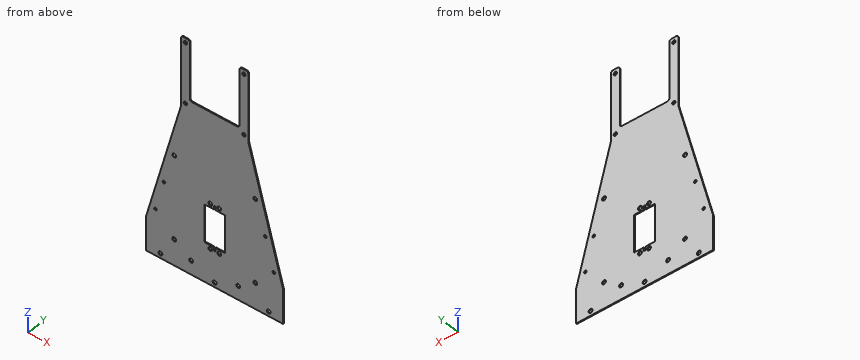
```python
from build123d import *

# Parameters (mm, degrees)
SKETCH26_R          = 1.875
SKETCH26_R_2        = 2.15
SKETCH26_R_3        = 1.45
BOSS_EXTRUDE6_DEPTH = 1


with BuildPart() as part:
    # Sketch26 → Boss-Extrude6 (new body)
    with BuildSketch(Plane(origin=(0, 0, 0), x_dir=(1, 0, 0), z_dir=(0, 1, 0))):
        with BuildLine():
            Line((76.013272408, 51.623832483), (76.013272408, 88.823544949))
            Line((76.013272408, 88.823544949), (-76.102081629, 88.823544949))
            Line((-76.102081629, 88.823544949), (-76.102081629, 51.776273242))
            Line((-76.102081629, 51.776273242), (-37.685470178, -85.312264175))
            ThreePointArc((-37.685470178, -85.312264175), (-37.546584556, -85.980512893), (-37.5, -86.661450073))
            Line((-37.5, -86.661450073), (-37.5, -159.216442532))
            ThreePointArc((-37.5, -159.216442532), (-36.767766953, -160.984209485), (-35, -161.716442532))
            Line((-35, -161.716442532), (-30, -161.716442532))
            ThreePointArc((-30, -161.716442532), (-28.232405329, -160.98438175), (-27.500000047, -159.216929795))
            Line((-27.500000047, -159.216929795), (-27.488305541, -99.215955269))
            ThreePointArc((-27.488305541, -99.215955269), (-26.755900259, -97.448503314), (-24.988305588, -96.716442532))
            Line((-24.988305588, -96.716442532), (24.988305588, -96.716442532))
            ThreePointArc((24.988305588, -96.716442532), (26.756072541, -97.448675579), (27.488305588, -99.216442532))
            Line((27.488305588, -99.216442532), (27.488305588, -159.216442532))
            ThreePointArc((27.488305588, -159.216442532), (28.220538635, -160.984209485), (29.988305588, -161.716442532))
            Line((29.988305588, -161.716442532), (34.988305588, -161.716442532))
            ThreePointArc((34.988305588, -161.716442532), (36.756072541, -160.984209485), (37.488305588, -159.216442532))
            Line((37.488305588, -159.216442532), (37.488305588, -86.69785128))
            ThreePointArc((37.488305588, -86.69785128), (37.534787412, -86.017661841), (37.673368657, -85.350118981))
            Line((37.673368657, -85.350118981), (75.502125614, 49.797698633))
            Line((75.502125614, 49.797698633), (76.013272408, 51.623832483))
        make_face()
        with Locations(Location((-32.5, -156.716442532, 0), (0, 0, 270))):
            Circle(SKETCH26_R, mode=Mode.SUBTRACT)
        with Locations(Location((-32.5, -91.716442532, 0), (0, 0, 270))):
            Circle(SKETCH26_R, mode=Mode.SUBTRACT)
        with Locations(Location((32.488305588, -156.716442532, 0), (0, 0, 270))):
            Circle(SKETCH26_R, mode=Mode.SUBTRACT)
        with Locations(Location((32.488305588, -91.716442532, 0), (0, 0, 270))):
            Circle(SKETCH26_R, mode=Mode.SUBTRACT)
        with Locations(Location((-44.91002895, -29.282587791, 0), (0, 0, 270))):
            Circle(SKETCH26_R_2, mode=Mode.SUBTRACT)
        with Locations(Location((-56.275133419, 5.22710987, 0), (0, 0, 270))):
            Circle(SKETCH26_R_3, mode=Mode.SUBTRACT)
        with Locations(Location((-4.91002895, 1.717412209, 0), (0, 0, 270))):
            Circle(SKETCH26_R_2, mode=Mode.SUBTRACT)
        with Locations(Location((-65.710275059, 38.931384113, 0), (0, 0, 270))):
            Circle(SKETCH26_R_3, mode=Mode.SUBTRACT)
        with Locations(Location((-60.263272408, 83.747616616, 0), (0, 0, 270))):
            Circle(SKETCH26_R_2, mode=Mode.SUBTRACT)
        with Locations(Location((-44.91002895, 60.717412209, 0), (0, 0, 270))):
            Circle(SKETCH26_R_2, mode=Mode.SUBTRACT)
        with Locations(Location((-4.91002895, 50.217412209, 0), (0, 0, 270))):
            Circle(SKETCH26_R_2, mode=Mode.SUBTRACT)
        with Locations(Location((-26.102081629, 73.823544949, 0), (0, 0, 270))):
            Circle(SKETCH26_R_2, mode=Mode.SUBTRACT)
        with Locations(Location((5.08997105, 1.717412209, 0), (0, 0, 270))):
            Circle(SKETCH26_R_2, mode=Mode.SUBTRACT)
        Polygon((11.577692982, 46.217412209), (11.577692982, 5.717412209), (1.08997105, 5.717412209), (1.08997105, 1.717412209), (-0.91002895, 1.717412209), (-0.91002895, 5.717412209), (-11.397750883, 5.717412209), (-11.397750883, 46.217412209), (-0.91002895, 46.217412209), (-0.91002895, 50.217412209), (1.08997105, 50.217412209), (1.08997105, 46.217412209), align=None, mode=Mode.SUBTRACT)
        with Locations(Location((45.08997105, -29.282587791, 0), (0, 0, 270))):
            Circle(SKETCH26_R_2, mode=Mode.SUBTRACT)
        with Locations(Location((56.276531408, 5.226515161, 0), (0, 0, 270))):
            Circle(SKETCH26_R_3, mode=Mode.SUBTRACT)
        with Locations(Location((5.08997105, 50.217412209, 0), (0, 0, 270))):
            Circle(SKETCH26_R_2, mode=Mode.SUBTRACT)
        with Locations(Location((0, 83.74802142, 0), (0, 0, 270))):
            Circle(SKETCH26_R_2, mode=Mode.SUBTRACT)
        with Locations(Location((26.102081629, 73.823544949, 0), (0, 0, 270))):
            Circle(SKETCH26_R_2, mode=Mode.SUBTRACT)
        with Locations(Location((65.7106575, 38.931073679, 0), (0, 0, 270))):
            Circle(SKETCH26_R_3, mode=Mode.SUBTRACT)
        with Locations(Location((45.08997105, 60.717412209, 0), (0, 0, 270))):
            Circle(SKETCH26_R_2, mode=Mode.SUBTRACT)
        with Locations(Location((59.999999999, 83.747618385, 0), (0, 0, 270))):
            Circle(SKETCH26_R_2, mode=Mode.SUBTRACT)
    extrude(amount=BOSS_EXTRUDE6_DEPTH)


solid = part.part
```
Here's how the part is built. I have some questions about the finished solid (model axes, mm). Coordinates: 2 decimals unless noted, no trailing zeros. Order: outer loops, then holes, each group sorted by start corner. A loop starts at its lowest first (then second) coordinate and runs counter-clockwise, first axis right, second up. Notation, with made-up numbers: (67, -12) -> (106, -12) arc R17 cw to (106, 11) -> close; hole circle Ø5 at (49.5, 50.5). An arc over 180 degrees is marked (long way). Return JSON: item names as keys, results as strings.
1) I'm going to push a flat-ended pin straight in: P1, Ø3.5, axis at x = 32.49, z = 156.72, coming from the +Y side. Where does the tip first touch, or does it pass through?
Conclusion:
{"P1": "passes through"}
2) If we section it at A-A on y = 0.35: State how many separate pieces and enclosed holes the cut face has, plus the area to 3 significant figures.
Conclusion:
{"separate pieces": "1", "enclosed holes": "22", "area": "22,200 mm²"}
3) If we section it at C-C on z = 51.5: List the corners of the cut face in (x, y) for me.
Conclusion:
{"outline": "(-47.16, 0) -> (47.15, 0) -> (47.15, 1) -> (-47.16, 1) -> close"}
4) If we section it at B-B on z = 11.5: List the corners of the cut face in (x, y) for me, plus the area to 3 significant figures.
Conclusion:
{"outline": "(-58.37, 0) -> (58.34, 0) -> (58.34, 1) -> (-58.37, 1) -> close", "area": "117 mm²"}
5) If I drill on probe 1 along X at (y, z) = (0.85, -49); probe 2 along X at (y, z) = (0.7, -5); probe 3 along X at (y, z) = (0.4, 95), over which ranges is the centre line in solid material (lowest first)?
Conclusion:
{"probe 1": "x = -75.32 to -6.68, -3.14 to -0.91, 1.09 to 3.32, 6.86 to 75.28", "probe 2": "x = -62.99 to -57.71, -54.84 to -0.91, 1.09 to 54.84, 57.71 to 62.96", "probe 3": "x = -37.5 to 37.49"}
